from build123d import *

# Parameters (mm, degrees)
SKETCH1_W           = 120
SKETCH1_H           = 140
BOSS_EXTRUDE1_DEPTH = 2
SKETCH2_R           = 1.525
SKETCH2_R_2         = 1.5
CUT_EXTRUDE1_DEPTH  = 2
SKETCH4_R           = 1.5
SKETCH4_R_2         = 1.55
SKETCH4_W           = 8
SKETCH4_H           = 60
CUT_EXTRUDE2_DEPTH  = 93.217135067
SKETCH5_R           = 1.5
CUT_EXTRUDE3_DEPTH  = 93.217135067


with BuildPart() as part:
    # Sketch1 → Boss-Extrude1 (new body)
    with BuildSketch(Plane(origin=(0, 0, 0), x_dir=(1, 0, 0), z_dir=(0, 1, 0))):
        Rectangle(SKETCH1_W, SKETCH1_H)
    extrude(amount=BOSS_EXTRUDE1_DEPTH)

    # Sketch2 → Cut-Extrude1 (cut)
    with BuildSketch(Plane(origin=(0, 2, 0), x_dir=(1, 0, 0), z_dir=(0, 1, 0))):
        with Locations(Location((-53, 64, 0), (0, 0, 270))):
            Circle(SKETCH2_R)
        with Locations(Location((-53, -64.8, 0), (0, 0, 270))):
            Circle(SKETCH2_R_2)
        with Locations(Location((53, 64, 0), (0, 0, 90))):
            Circle(SKETCH2_R)
        with Locations(Location((53, -64.8, 0), (0, 0, 90))):
            Circle(SKETCH2_R_2)
    extrude(amount=-CUT_EXTRUDE1_DEPTH, mode=Mode.SUBTRACT)

    # Sketch4 → Cut-Extrude2 (cut, through all)
    with BuildSketch(Plane(origin=(0, 2, 0), x_dir=(1, 0, 0), z_dir=(0, 1, 0))):
        with Locations(Location((-25, 63, 0), (0, 0, 270))):
            Circle(SKETCH4_R)
        with Locations(Location((-25, -12.13, 0), (0, 0, 270))):
            Circle(SKETCH4_R)
        with Locations(Location((23.33, -12.13, 0), (0, 0, 270))):
            Circle(SKETCH4_R_2)
        with Locations((-39, 30)):
            Rectangle(SKETCH4_W, SKETCH4_H)
        with Locations((39, 30)):
            Rectangle(SKETCH4_W, SKETCH4_H)
    extrude(amount=-CUT_EXTRUDE2_DEPTH, mode=Mode.SUBTRACT)

    # Sketch5 → Cut-Extrude3 (cut, through all)
    with BuildSketch(Plane(origin=(0, 2, 0), x_dir=(1, 0, 0), z_dir=(0, 1, 0))):
        with Locations(Location((-54, -55, 0), (0, 0, 270))):
            Circle(SKETCH5_R)
        with Locations(Location((-28.82, -55, 0), (0, 0, 270))):
            Circle(SKETCH5_R)
        with Locations(Location((-54, -31.9, 0), (0, 0, 270))):
            Circle(SKETCH5_R)
    extrude(amount=-CUT_EXTRUDE3_DEPTH, mode=Mode.SUBTRACT)


solid = part.part
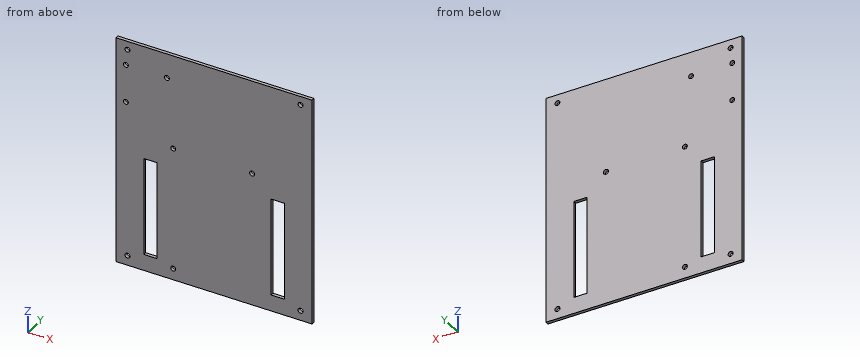
Read the model definition and answer for the solid it produces. Units are mm, in the model's axes. Coordinates: 2 decimals unless noted, no trailing zeros. Loops run counter-clockwise (first coordinate to the right, second up) from the corner with the lowest first, then second, coordinate; pieces in that order, holes last. Notation, with made-up numbers: (16.25, -20.5) -> (60.25, -20.5) arc R29 ccw to (60.25, 14.5) -> close; hole circle Ø3 at (58.5, 6). An arc over 180 degrees is marked (long way). Answer in a Markdown table with one row per item.
Item 1: A cutting plane is placed at C-C on z = -58. Determine the outline of the cut face in (x, y), plus the area to 3 significant figures.
Returned:
| item | result |
|---|---|
| outline | (-60, 0) -> (-43, 0) -> (-43, 2) -> (-60, 2) -> close; (-35, 0) -> (35, 0) -> (35, 2) -> (-35, 2) -> close; (43, 0) -> (60, 0) -> (60, 2) -> (43, 2) -> close |
| area | 208 mm^2 |
Item 2: A cutting plane is placed at D-D on z = 31.9. Determine the outline of the cut face in (x, y), plus the area to 3 significant figures.
Returned:
| item | result |
|---|---|
| outline | (-60, 0) -> (-55.5, 0) -> (-55.5, 2) -> (-60, 2) -> close; (-52.5, 0) -> (60, 0) -> (60, 2) -> (-52.5, 2) -> close |
| area | 234 mm^2 |
Item 3: A cutting plane is placed at B-B on y = 1.1. Give the number of separate pieces and of enclosed holes in the cut face, plus the area to 3 significant figures.
Returned:
| item | result |
|---|---|
| separate pieces | 1 |
| enclosed holes | 12 |
| area | 15,800 mm^2 |
Item 4: Straight lines are drawn through the part: line 1 along X through (y, z) = (1.45, 12.13); line 2 along X through (y, z) = (1, -58.5); line 3 along Z through (x, y) = (53, 1.4) (3 decimals). For each, find the intervals that lie inside material, in ascending order. Write a range as [from, to].
Returned:
| item | result |
|---|---|
| line 1 | x = [-60, -26.5], [-23.5, 21.78], [24.88, 60] |
| line 2 | x = [-60, -43], [-35, 35], [43, 60] |
| line 3 | z = [-70, -65.525], [-62.475, 63.3], [66.3, 70] |
Item 5: A cutting plane is placed at A-A on x = 23.33. Determine the outline of the cut face in (y, z).
Returned:
| item | result |
|---|---|
| outline | (0, -70) -> (2, -70) -> (2, 10.58) -> (0, 10.58) -> close; (0, 13.68) -> (2, 13.68) -> (2, 70) -> (0, 70) -> close |
